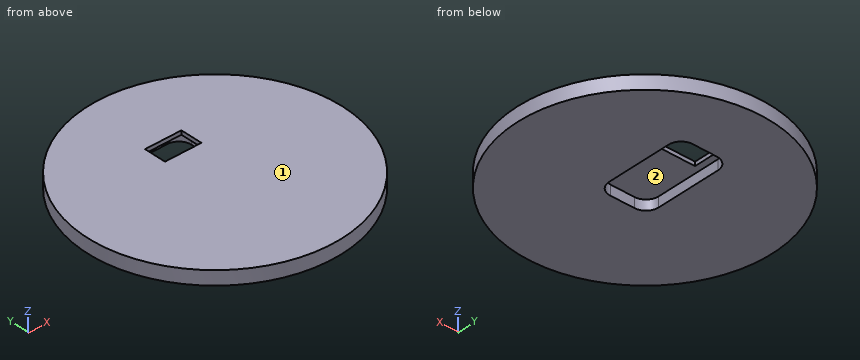
```python
from build123d import *

# Parameters (mm, degrees)
SKETCH1_R           = 63.76
BOSS_EXTRUDE1_DEPTH = 7
SKETCH4_W           = 24.8
SKETCH4_H           = 45.33
CUT_EXTRUDE1_DEPTH  = 5
FILLET1_R           = 6.35
CUT_EXTRUDE2_REACH  = 92.309
SKETCH5_W           = 18.224025504
SKETCH5_H           = 11.004820717


with BuildPart() as part:
    # Sketch1 → Boss-Extrude1 (new body)
    with BuildSketch(Plane.XY):
        Circle(SKETCH1_R)
    extrude(amount=BOSS_EXTRUDE1_DEPTH)

    # Sketch4 → Cut-Extrude1 (cut)
    with BuildSketch(Plane(origin=(0, 0, 0), x_dir=(-1, 0, 0), z_dir=(0, 0, -1))):
        with Locations((0, 10.245)):
            Rectangle(SKETCH4_W, SKETCH4_H)
    extrude(amount=-CUT_EXTRUDE1_DEPTH, mode=Mode.SUBTRACT)

    # Fillet1
    fillet1_edges = [part.edges().sort_by_distance(p)[0] for p in [
        (12.4, -12.42, 2.5),
        (12.4, 32.91, 2.5),
        (-12.4, 32.91, 2.5),
        (-12.4, -12.42, 2.5),
    ]]
    fillet(fillet1_edges, radius=FILLET1_R)

    # Sketch5 → Cut-Extrude2 (cut, up to next)
    with BuildSketch(Plane(origin=(0, 0, 5), x_dir=(-1, 0, 0), z_dir=(0, 0, -1)), mode=Mode.PRIVATE) as cut_extrude2_sk1:
        with Locations((0, 23.06297221)):
            Rectangle(SKETCH5_W, SKETCH5_H)
    cut_extrude2_tool1 = extrude(cut_extrude2_sk1.sketch, amount=-CUT_EXTRUDE2_REACH, mode=Mode.PRIVATE) & part.part
    add(cut_extrude2_tool1.solids().sort_by_distance((0, 23.062972, 5))[0], mode=Mode.SUBTRACT)


solid = part.part
```
Could you check a few things on this model? Use its own coordinates, in mm. Face numbers are marked on the shaded views. Coordinates: 2 decimals unless noted, no trailing zeros. Loops run counter-clockwise (first coordinate to the right, second up) from the corner with the lowest first, then second, coordinate; pieces in that order, holes last. Notation, with made-up numbers: M 33.25,61 L 55.25,61 A20 cw 55.25,75 Z; hole C 24,-4.75 d5. An arc over 180 degrees is marked long. Put each result on its own line as item: value. Start each with the question number.
(1) Thinking about a two-plate mould opening in X: for the marked faces 1 and 2, which applies, pulls with the +X half, pulls with the -X half, needs draft (parallel to the pull), parting line crosses it, or undercut?
(2) Suppose I cut it at D-D on x = 49.5. Please give me the cut outline in (y, z).
(3) Suppose I cut it at C-C on y = 0. Please give me the cut outline in (x, z).
(4) Suppose I cut it at A-A on x = 0. Please give me the cut outline in (y, z).
(5) Will these pins go through, and if not, where does the flat tip stop? P1, Ø2.5, axis at y = 17.5, z = 2, coming from the +X side; P2, Ø1, axis at x = 28, z = 5.5, coming from the +Y side; P3, Ø4, axis at x = 7, z = 5.5, coming from the -Y side.
(6) I need wall thicknesses on line 1 (X direction, y = 14.5, z = 3.5); line 2 (X direction, y = 54.5, z = 4.5); line 3 (Y direction, x = -50, z = 5.25). Which ranges of each line are inside material? Lowest first, please. Write a range as from..to.
(7) Suppose I cut it at B-B on z = 3.5. Please give me the cut outline in (x, y), then the cut area to 3 significant figures.
Solutions:
1. face 1: needs draft
1. face 2: undercut
2. outline: M -40.19,0 L 40.19,0 L 40.19,7 L -40.19,7 Z
3. outline: M -63.76,0 L -12.4,0 L -12.4,5 L 12.4,5 L 12.4,0 L 63.76,0 L 63.76,7 L -63.76,7 Z
4. outline: M -63.76,0 L -12.42,0 L -12.42,5 L 17.56,5 L 17.56,7 L -63.76,7 Z; M 28.57,5 L 32.91,5 L 32.91,0 L 63.76,0 L 63.76,7 L 28.57,7 Z
5. P1: stops at x = 61.65
5. P2: stops at y = 57.52
5. P3: stops at y = -63.56
6. line 1: x = -62.09..-12.4, 12.4..62.09
6. line 2: x = -33.09..33.09
6. line 3: y = -39.56..39.56
7. outline: C 0,0 d127.52; hole M -12.4,-6.07 A6.35 ccw -6.05,-12.42 L 6.05,-12.42 A6.35 ccw 12.4,-6.07 L 12.4,26.56 A6.35 ccw 6.05,32.91 L -6.05,32.91 A6.35 ccw -12.4,26.56 Z
7. area: 11,700 mm2
